Model file for the job. Use its own axes, mm. A direction names the side the tool comes from. Round coordinates to 2 decimals unless told otherwise and drop trailing zeros. Write each loop counter-clockwise with the first axis right and the second up, starting at its lowest first coordinate (ties: lowest second). Pieces come first, ordered by that corner, then holes. Notation, with made-up numbers: (45.5, 75.5) - (87.5, 75.5) arc R7 ccw to (87.5, 84.5) - close; hole circle Ø6 at (-29, 14). An arc over 180 degrees is marked (long way). One line per item, written item: value.
from build123d import *

# Parameters (mm, degrees)
SKETCH1_R           = 4.1275
BOSS_EXTRUDE1_DEPTH = 1.27


with BuildPart() as part:
    # Sketch1 → Boss-Extrude1 (new body)
    with BuildSketch(Plane.XY):
        with BuildLine():
            Line((-0.66010495, -6.301124731), (-0.946700317, -9.036861149))
            ThreePointArc((-0.946700317, -9.036861149), (-0.007173127, -9.086311103), (0.932430967, -9.038344617))
            Line((0.932430967, -9.038344617), (0.650155372, -6.302159107))
            ThreePointArc((0.650155372, -6.302159107), (1.953052705, -6.027063676), (3.169672067, -5.485716945))
            Line((3.169672067, -5.485716945), (4.545837066, -7.86743073))
            ThreePointArc((4.545837066, -7.86743073), (5.334996482, -7.355196357), (6.066958169, -6.764105225))
            Line((6.066958169, -6.764105225), (4.230302926, -4.716402079))
            ThreePointArc((4.230302926, -4.716402079), (5.122671972, -3.728021363), (5.788742087, -2.57495174))
            Line((5.788742087, -2.57495174), (8.302019196, -3.692909176))
            ThreePointArc((8.302019196, -3.692909176), (8.639378766, -2.814646597), (8.884113559, -1.906207541))
            Line((8.884113559, -1.906207541), (6.194618544, -1.329139762))
            ThreePointArc((6.194618544, -1.329139762), (6.335604659, -0.005001601), (6.196709383, 1.319357511))
            Line((6.196709383, 1.319357511), (8.887112169, 1.892178166))
            ThreePointArc((8.887112169, 1.892178166), (8.643812002, 2.801002498), (8.30783953, 3.679796635))
            Line((8.30783953, 3.679796635), (5.792800426, 2.565808769))
            ThreePointArc((5.792800426, 2.565808769), (5.128551706, 3.719928603), (4.237744312, 4.709717036))
            Line((4.237744312, 4.709717036), (6.077630355, 6.754517761))
            ThreePointArc((6.077630355, 6.754517761), (5.346602846, 7.34676384), (4.558253173, 7.860243567))
            Line((4.558253173, 7.860243567), (3.178329436, 5.480705558))
            ThreePointArc((3.178329436, 5.480705558), (1.962566314, 6.023972516), (0.66010495, 6.301124731))
            Line((0.66010495, 6.301124731), (0.946700317, 9.036861149))
            ThreePointArc((0.946700317, 9.036861149), (0.007173127, 9.086311103), (-0.932430967, 9.038344617))
            Line((-0.932430967, 9.038344617), (-0.650155372, 6.302159107))
            ThreePointArc((-0.650155372, 6.302159107), (-1.953052705, 6.027063676), (-3.169672067, 5.485716945))
            Line((-3.169672067, 5.485716945), (-4.545837066, 7.86743073))
            ThreePointArc((-4.545837066, 7.86743073), (-5.334996482, 7.355196357), (-6.066958169, 6.764105225))
            Line((-6.066958169, 6.764105225), (-4.230302926, 4.716402079))
            ThreePointArc((-4.230302926, 4.716402079), (-5.122671972, 3.728021363), (-5.788742087, 2.57495174))
            Line((-5.788742087, 2.57495174), (-8.302019196, 3.692909176))
            ThreePointArc((-8.302019196, 3.692909176), (-8.639378766, 2.814646597), (-8.884113559, 1.906207541))
            Line((-8.884113559, 1.906207541), (-6.194618544, 1.329139762))
            ThreePointArc((-6.194618544, 1.329139762), (-6.335604659, 0.005001601), (-6.196709383, -1.319357511))
            Line((-6.196709383, -1.319357511), (-8.887112169, -1.892178166))
            ThreePointArc((-8.887112169, -1.892178166), (-8.643812002, -2.801002498), (-8.30783953, -3.679796635))
            Line((-8.30783953, -3.679796635), (-5.792800426, -2.565808769))
            ThreePointArc((-5.792800426, -2.565808769), (-5.128551706, -3.719928603), (-4.237744312, -4.709717036))
            Line((-4.237744312, -4.709717036), (-6.077630355, -6.754517761))
            ThreePointArc((-6.077630355, -6.754517761), (-5.346602846, -7.34676384), (-4.558253173, -7.860243567))
            Line((-4.558253173, -7.860243567), (-3.178329436, -5.480705558))
            ThreePointArc((-3.178329436, -5.480705558), (-1.962566314, -6.023972516), (-0.66010495, -6.301124731))
        make_face()
        Circle(SKETCH1_R, mode=Mode.SUBTRACT)
    extrude(amount=BOSS_EXTRUDE1_DEPTH)


solid = part.part
1. Tool access for faces 4 (the face through (0.02, 9.086, 0.626)), 5 (the face through (5.139, 3.705, 0.626)), 6 (the face through (-7.558, 1.622, 0.626)), 7 (the face through (5.2, -5.8, 0.6)), 8 (the face through (8.635, -2.827, 0.626)): list every direction of +Z, -Z, +X, -X, +Y, -Y with a clear straight run to the whole face (end or side of a thin tool).
Report:
face 4: +Z, -Z, +Y
face 5: +Z, -Z
face 6: +Z, -Z, -X
face 7: +Z, -Z, +X
face 8: +Z, -Z, +X, -Y
2. Drop flat-ended pins along their axis: pin 1 (10 mm diameter, centred on x = -2.5, y = 5, fed in from -Z); pin 2 (1.5 mm diameter, centred on x = 2.5, y = 2, fed in from +Z). Give the stop position or say it passes through.
Report:
pin 1: z = 0
pin 2: through
3. Wall check: probe 1 along Y at (x, z) = (0, 0.55); probe 2 along Y at (x, z) = (-4.75, 0.2); probe 3 along X at (y, z) = (-5.75, 1.2). Give the ranges that are in metal, low to high. Write a range as [from, to].
Report:
probe 1: [-9.09, -4.13], [4.13, 9.09]
probe 2: [-7.75, -5.28], [-4.19, 4.19], [5.3, 7.75]
probe 3: [-5.17, -3.33], [-2.66, 2.66], [3.32, 5.16]
4. Mould opens along X. For faces 1 (the face through (5.112, -3.743, 0.626)), 2 (the face through (-5.357, -7.339, 0.626)), 3 (the face through (5.145, 5.718, 0.626)) say: released by +X, released by -X, zero draft, split by the parting line, or undercut.
Report:
face 1: undercut
face 2: released by -X
face 3: released by +X
5. Band-saw the part on B-B on x = 0. Write the cut outline in (y, z).
Report:
outline: (-9.09, 0) - (-4.13, 0) - (-4.13, 1.27) - (-9.09, 1.27) - close; (4.13, 0) - (9.09, 0) - (9.09, 1.27) - (4.13, 1.27) - close
6. Band-saw the part on C-C on y = -7.25. Write the cut outline in (x, z), plus the area to 3 significant figures.
Report:
outline: (-5.48, 0) - (-4.2, 0) - (-4.2, 1.27) - (-5.48, 1.27) - close; (-0.76, 0) - (0.75, 0) - (0.75, 1.27) - (-0.76, 1.27) - close; (4.19, 0) - (5.48, 0) - (5.48, 1.27) - (4.19, 1.27) - close
area: 5.17 mm²
7. Band-saw the part on D-D on x = -5.5. Write the cut outline in (y, z), plus the area to 3 significant figures.
Report:
outline: (-7.23, 0) - (-6.11, 0) - (-6.11, 1.27) - (-7.23, 1.27) - close; (-3.14, 0) - (3.14, 0) - (3.14, 1.27) - (-3.14, 1.27) - close; (6.13, 0) - (7.23, 0) - (7.23, 1.27) - (6.13, 1.27) - close
area: 10.8 mm²
8. Band-saw the part on A-A on y = 0. Write the cut outline in (x, z).
Report:
outline: (-6.34, 0) - (-4.13, 0) - (-4.13, 1.27) - (-6.34, 1.27) - close; (4.13, 0) - (6.34, 0) - (6.34, 1.27) - (4.13, 1.27) - close
